Job drawing, mm, ordinate dimensions from the low corner. One solid piece. A direction names the side the tool comes from. Give positions to 0.01 mm unless a question says otherwise; leave off trailing zeros. Order: outer loops, then holes, each group sorted by start corner. A loop starts at its lowest first (then second) coordinate and runs counter-clockwise, first axis right, second up. Notation, with made-up numbers: M 71,62 L 112,62 A15 ccw 112,68 Z; hole C -14.75,68 d3. An arc over 180 degrees is marked long. One line per question, with ' | ' between items.
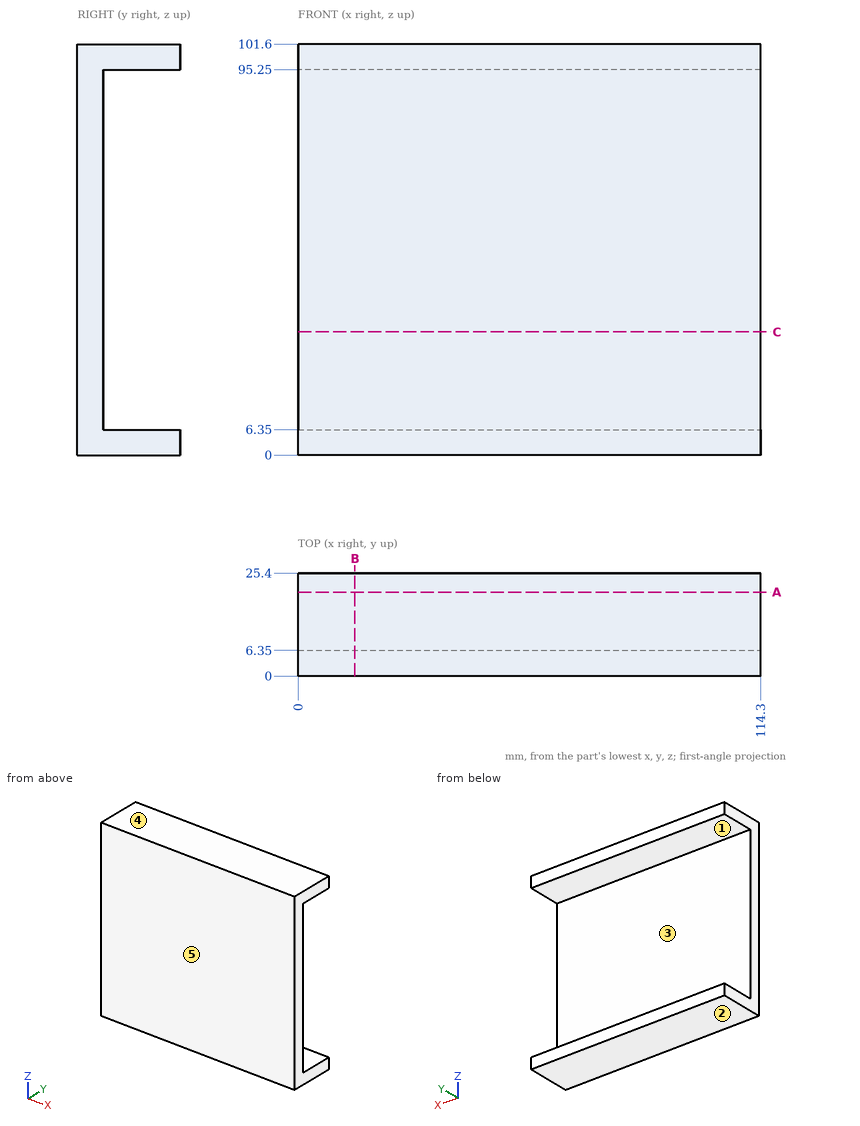
1. Probe L1, parallel to Z at x = 104, y = 17.5; L2, parallel to Y at x = 107.5, z = 53.5. List the from-to ranges inside material, lowest first. Write a range as from..to.
Worked out:
L1: z = 0..6.35, 95.25..101.6 | L2: y = 0..6.35
2. Tool access for the marked faces 1 and 2: list every direction of +Z, -Z, +X, -X, +Y, -Y with a clear straight run to the whole face (end or side of a thin tool).
Worked out:
face 1: +X, -X, +Y | face 2: -Z, +X, -X, +Y, -Y
3. Slice it at C-C on z = 30.5. Give the cut face in (x, y).
Worked out:
outline: M 0,0 L 114.3,0 L 114.3,6.35 L 0,6.35 Z
4. Mould opens along Z. For the marked faces 3, 4 and 5 say: released by +Z, released by -Z, zero draft, split by the parting line, or undercut.
Worked out:
face 3: undercut | face 4: released by +Z | face 5: zero draft
5. Slice it at A-A on y = 20.75. Give the cut face in (x, z).
Worked out:
outline: M 0,0 L 114.3,0 L 114.3,6.35 L 0,6.35 Z; M 0,95.25 L 114.3,95.25 L 114.3,101.6 L 0,101.6 Z
6. Slice it at B-B on x = 14. Give the cut face in (y, z), then the cut area to 3 significant figures.
Worked out:
outline: M 0,0 L 25.4,0 L 25.4,6.35 L 6.35,6.35 L 6.35,95.25 L 25.4,95.25 L 25.4,101.6 L 0,101.6 Z | area: 887 mm2
